Read the model definition and answer for the solid it produces. Units are mm, in the model's axes. Face numbers are marked on the shaded views. A direction names the side the tool comes from. Give positions to 0.01 mm unless a question says otherwise; leave off trailing zeros. Write each loop counter-clockwise with the first axis right and the second up, starting at its lowest first coordinate (ties: lowest second). Pieces come first, ordered by that corner, then holes. Notation, with made-up numbers: (12.25, 22.25) - (20.25, 22.25) arc R24 ccw to (20.25, 35.25) - close; hole circle Ø1 at (7.5, 35). An arc over 180 degrees is marked (long way). Answer as CSV lines item,"result".
```python
from build123d import *

# Parameters (mm, degrees)
ESQUISSE1_W             = 10
ESQUISSE1_H             = 5
BOSS_EXTRU_1_DEPTH      = 8
ESQUISSE2_W             = 6.6
ESQUISSE2_H             = 0.8
ENL_V_MAT_EXTRU_1_DEPTH = 8
ENL_V_MAT_EXTRU_2_DEPTH = 6.5
ESQUISSE5_W             = 6
ESQUISSE5_H             = 0.5
ENL_V_MAT_EXTRU_3_DEPTH = 1
ESQUISSE6_W             = 5.6
ESQUISSE6_H             = 0.5
ENL_V_MAT_EXTRU_4_DEPTH = 3
ESQUISSE7_W             = 0.8
ESQUISSE7_H             = 1
ENL_V_MAT_EXTRU_5_DEPTH = 10
ESQUISSE8_W             = 6.8
ESQUISSE8_H             = 4.2
ENL_V_MAT_EXTRU_6_DEPTH = 1
BOSS_EXTRU_2_DEPTH      = 6.8
BOSS_EXTRU_3_DEPTH      = 2
BOSS_EXTRU_3_DEPTH_BACK = 2
ESQUISSE12_W            = 0.5
ESQUISSE12_H            = 4.2
BOSS_EXTRU_4_DEPTH      = 1
CHANFREIN1_SIZE         = 0.15
BOSS_EXTRU_5_DEPTH      = 3.2
BOSS_EXTRU_5_DEPTH_BACK = 5
ESQUISSE13_W            = 0.425
ESQUISSE13_H            = 0.45
CHANFREIN2_SIZE         = 0.1


with BuildPart() as part:
    # Esquisse1 → Boss.-Extru.1 (new body)
    with BuildSketch(Plane(origin=(0, 0, 0), x_dir=(1, 0, 0), z_dir=(0, 1, 0))):
        with Locations((5, 2.5)):
            Rectangle(ESQUISSE1_W, ESQUISSE1_H)
    extrude(amount=BOSS_EXTRU_1_DEPTH)

    # Esquisse2 → Enlèv. mat.-Extru.1 (cut)
    with BuildSketch(Plane(origin=(0, 8, 0), x_dir=(1, 0, 0), z_dir=(0, 1, 0))):
        with Locations((5, 0.4)):
            Rectangle(ESQUISSE2_W, ESQUISSE2_H)
    extrude(amount=-ENL_V_MAT_EXTRU_1_DEPTH, mode=Mode.SUBTRACT)

    # Esquisse4 → Enlèv. mat.-Extru.2 (cut)
    with BuildSketch(Plane(origin=(0, 8, 0), x_dir=(1, 0, 0), z_dir=(0, 1, 0))):
        Polygon((0.5, 0.5), (1.2, 0.5), (1.2, 1.3), (8.8, 1.3), (8.8, 0.5), (9.5, 0.5), (9.5, 4.5), (0.5, 4.5), align=None)
    extrude(amount=-ENL_V_MAT_EXTRU_2_DEPTH, mode=Mode.SUBTRACT)

    # Esquisse5 → Enlèv. mat.-Extru.3 (cut)
    with BuildSketch(Plane(origin=(0, 8, 0), x_dir=(1, 0, 0), z_dir=(0, 1, 0))):
        with Locations((5, 4.75)):
            Rectangle(ESQUISSE5_W, ESQUISSE5_H)
    extrude(amount=-ENL_V_MAT_EXTRU_3_DEPTH, mode=Mode.SUBTRACT)

    # Esquisse6 → Enlèv. mat.-Extru.4 (cut)
    with BuildSketch(Plane(origin=(0, 8, 0), x_dir=(1, 0, 0), z_dir=(0, 1, 0))):
        with Locations((5, 1.05)):
            Rectangle(ESQUISSE6_W, ESQUISSE6_H)
    extrude(amount=-ENL_V_MAT_EXTRU_4_DEPTH, mode=Mode.SUBTRACT)

    # Esquisse7 → Enlèv. mat.-Extru.5 (cut)
    with BuildSketch(Plane(origin=(10, 0, 0), x_dir=(0, 0, -1), z_dir=(1, 0, 0))):
        with Locations((0.4, 0.5)):
            Rectangle(ESQUISSE7_W, ESQUISSE7_H)
    extrude(amount=-ENL_V_MAT_EXTRU_5_DEPTH, mode=Mode.SUBTRACT)

    # Esquisse8 → Enlèv. mat.-Extru.6 (cut)
    with BuildSketch(Plane.XZ):
        with Locations((5, -2.9)):
            Rectangle(ESQUISSE8_W, ESQUISSE8_H)
    extrude(amount=-ENL_V_MAT_EXTRU_6_DEPTH, mode=Mode.SUBTRACT)

    # Esquisse9 → Boss.-Extru.2 (add)
    with BuildSketch(Plane(origin=(1.6, 0, 0), x_dir=(0, 0, -1), z_dir=(1, 0, 0))):
        Polygon((4.7, 1), (3.9, 0.2), (1.9, 0.2), (1.1, 1), align=None)
    extrude(amount=BOSS_EXTRU_2_DEPTH)

    # Esquisse11 → Boss.-Extru.3 (add, two sides: drawn at the far end of the back side and taken through both)
    with BuildSketch(Plane(origin=(5, 0, 0), x_dir=(0, 0, -1), z_dir=(1, 0, 0)).offset(-BOSS_EXTRU_3_DEPTH_BACK)):
        Polygon((0.8, 5), (0.1, 3.4), (0.8, 3.4), align=None)
    extrude(amount=BOSS_EXTRU_3_DEPTH + BOSS_EXTRU_3_DEPTH_BACK)

    # Esquisse12 → Boss.-Extru.4 (add)
    with BuildSketch(Plane(origin=(0, 1, 0), x_dir=(1, 0, 0), z_dir=(0, 1, 0))):
        with Locations((5, 2.9)):
            Rectangle(ESQUISSE12_W, ESQUISSE12_H)
        with Locations((3.175, 2.9)):
            Rectangle(ESQUISSE12_W, ESQUISSE12_H)
        with Locations((6.825, 2.9)):
            Rectangle(ESQUISSE12_W, ESQUISSE12_H)
    extrude(amount=-BOSS_EXTRU_4_DEPTH)

    # Chanfrein1
    chanfrein1_edges = [part.edges().sort_by_distance(p)[0] for p in [
        (2.2, 8, -1.05),
        (7.8, 8, -1.05),
    ]]
    chamfer(chanfrein1_edges, length=CHANFREIN1_SIZE)

    # Esquisse13 → Boss.-Extru.5 (add, two sides: drawn at the far end of the back side and taken through both)
    with BuildSketch(Plane.XZ.offset(-0.2).offset(-BOSS_EXTRU_5_DEPTH_BACK)):
        with Locations((2.2625, -2.9)):
            Rectangle(ESQUISSE13_W, ESQUISSE13_H)
        with Locations((4.0875, -2.9)):
            Rectangle(ESQUISSE13_W, ESQUISSE13_H)
        with Locations((5.9125, -2.9)):
            Rectangle(ESQUISSE13_W, ESQUISSE13_H)
        with Locations((7.7375, -2.9)):
            Rectangle(ESQUISSE13_W, ESQUISSE13_H)
    extrude(amount=BOSS_EXTRU_5_DEPTH + BOSS_EXTRU_5_DEPTH_BACK)

    # Chanfrein2
    chanfrein2_edges = [part.edges().sort_by_distance(p)[0] for p in [
        (2.05, 5.2, -2.9),
        (2.2625, 5.2, -2.675),
        (2.475, 5.2, -2.9),
        (2.2625, 5.2, -3.125),
        (2.05, -3, -2.9),
        (2.2625, -3, -3.125),
        (2.475, -3, -2.9),
        (2.2625, -3, -2.675),
        (4.3, 5.2, -2.9),
        (4.0875, 5.2, -3.125),
        (3.875, 5.2, -2.9),
        (4.0875, 5.2, -2.675),
        (4.3, -3, -2.9),
        (4.0875, -3, -2.675),
        (3.875, -3, -2.9),
        (4.0875, -3, -3.125),
        (5.7, 5.2, -2.9),
        (5.9125, 5.2, -2.675),
        (6.125, 5.2, -2.9),
        (5.9125, 5.2, -3.125),
        (5.7, -3, -2.9),
        (5.9125, -3, -3.125),
        (6.125, -3, -2.9),
        (5.9125, -3, -2.675),
        (7.7375, 5.2, -2.675),
        (7.95, 5.2, -2.9),
        (7.7375, 5.2, -3.125),
        (7.525, 5.2, -2.9),
        (7.7375, -3, -2.675),
        (7.525, -3, -2.9),
        (7.7375, -3, -3.125),
        (7.95, -3, -2.9),
    ]]
    chamfer(chanfrein2_edges, length=CHANFREIN2_SIZE)


solid = part.part
```
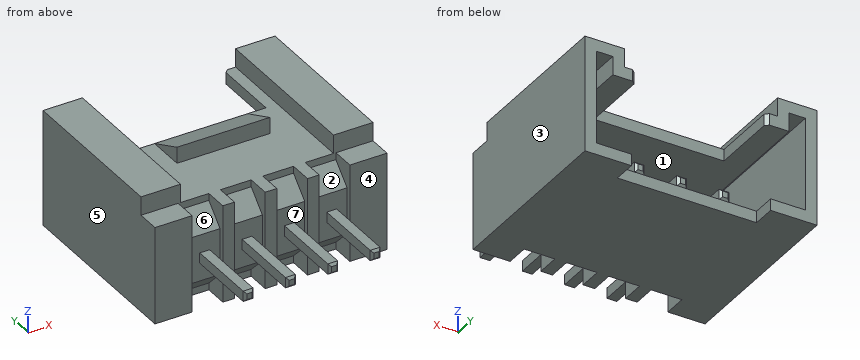
(1) A cutting plane is placed at C-C (z = -2.35). Write down the section's boundary in (x, y) (3 decimals).
Worked out:
outline,"(0, 0) - (1.6, 0) - (1.6, 0.2) - (2.925, 0.2) - (2.925, 0) - (3.425, 0) - (3.425, 0.2) - (4.75, 0.2) - (4.75, 0) - (5.25, 0) - (5.25, 0.2) - (6.575, 0.2) - (6.575, 0) - (7.075, 0) - (7.075, 0.2) - (8.4, 0.2) - (8.4, 0) - (10, 0) - (10, 8) - (9.5, 8) - (9.5, 1.5) - (0.5, 1.5) - (0.5, 8) - (0, 8) - close"
(2) Each of these flat-tipped pins is pushed along its axis until it touches: P1, Ø2, axis at x = 7.5, z = -1, coming from the -Y side; P2, Ø0.5, axis at y = -1.5, z = -3, coming from the -X side; P3, Ø0.5, axis at x = 6, y = 4, coming from the +Z side. Where does it stop, or does it pass through?
Worked out:
P1,"stops at y = 0"
P2,"stops at x = 2.05"
P3,"stops at z = -0.25"
(3) A cutting plane is placed at B-B (x = 9). Write down the section's boundary in (y, z).
Worked out:
outline,"(0, -5) - (8, -5) - (8, -4.5) - (1.5, -4.5) - (1.5, -0.5) - (8, -0.5) - (8, 0) - (1, 0) - (1, -0.8) - (0, -0.8) - close"
(4) A cutting plane is placed at D-D (y = 5.5). Write down the section's boundary in (x, z).
Worked out:
outline,"(0, -5) - (10, -5) - (10, 0) - (8.3, 0) - (8.3, -0.8) - (7.8, -0.8) - (7.8, -1.3) - (8.8, -1.3) - (8.8, -0.5) - (9.5, -0.5) - (9.5, -4.5) - (0.5, -4.5) - (0.5, -0.5) - (1.2, -0.5) - (1.2, -1.3) - (2.2, -1.3) - (2.2, -0.8) - (1.7, -0.8) - (1.7, 0) - (0, 0) - close"
(5) Find the intervals of material crossed by L1, parallel to Z at x = 5.25, y = 2.25; L2, parallel to Z at x = 4, y = 3.5 (3 decimals); L3, parallel to Z at x = 8.75, y = 3.75, in increasing order.
Worked out:
L1,"z = -5 to -4.5, -1.3 to -0.8"
L2,"z = -5 to -4.5, -3.125 to -2.675, -1.3 to -0.144"
L3,"z = -5 to -4.5, -1.3 to 0"
(6) A cutting plane is placed at A-A (y = -1.5). Write down the section's boundary in (x, z) (3 decimals).
Worked out:
outline,"(2.05, -3.125) - (2.475, -3.125) - (2.475, -2.675) - (2.05, -2.675) - close; (3.875, -3.125) - (4.3, -3.125) - (4.3, -2.675) - (3.875, -2.675) - close; (5.7, -3.125) - (6.125, -3.125) - (6.125, -2.675) - (5.7, -2.675) - close; (7.525, -3.125) - (7.95, -3.125) - (7.95, -2.675) - (7.525, -2.675) - close"
(7) The mould has two halves that part along X. Classify the marked faces 4, 5, 6 and 7: +X half, -X half, draft (parallel to the pull), parting line (faces both ways), or undercut.
Worked out:
face 4,"draft"
face 5,"-X half"
face 6,"undercut"
face 7,"undercut"
(8) For the marked faces 1, 2 and 3, determine the directions among +Z, -Z, +X, -X, +Y, -Y from which every point of the face is accessible in a straight line to the end or side of a thin tool.
Worked out:
face 1,"+Y"
face 2,"+Z, -Y"
face 3,"+Z, -Z, +X, +Y, -Y"
